from build123d import *
from build123d.topology import SkipClean

# Parameters (mm, degrees)
EXTRUDE_1_DEPTH          = 3
EXTRUDE_2_DEPTH          = 15
PATTERN_CIRCULAR_1_COUNT = 3
CUT_EXTRUDE_1_DEPTH      = 70.054326439


with BuildPart() as part:
    # Эскиз1 → Повернуть1 (revolve)
    with BuildSketch(Plane.XY, mode=Mode.PRIVATE) as revolve_1_sk:
        Polygon((0, 8), (0, 26.5), (10, 26.5), (10, 14), (40, 14), (40, 8), align=None)
    revolve(revolve_1_sk.sketch.rotate(Axis((0, 0, 0), (1, 0, 0)), 90), axis=Axis((0, 0, 0), (1, 0, 0)))

    # Эскиз2 → Бобышка-Вытянуть1 (add)
    with BuildSketch(Plane.ZY):
        with BuildLine():
            Line((22.9496732, 13.25), (14, 8.082903769))
            Line((14, 8.082903769), (14, -8.082903769))
            Line((14, -8.082903769), (22.9496732, -13.25))
            ThreePointArc((22.9496732, -13.25), (26.5, 0), (22.9496732, 13.25))
        make_face()
    extrude_1 = extrude(amount=EXTRUDE_1_DEPTH)

    # Эскиз3 → Бобышка-Вытянуть2 (add)
    with BuildSketch(Plane.ZY.offset(3)):
        with BuildLine():
            Line((25.037468802, 8.681886661), (14, 2.309401077))
            Line((14, 2.309401077), (14, -2.309401077))
            Line((14, -2.309401077), (25.037468802, -8.681886661))
            ThreePointArc((25.037468802, -8.681886661), (26.5, 0), (25.037468802, 8.681886661))
        make_face()
    extrude_2 = extrude(amount=EXTRUDE_2_DEPTH)

    # Круговой массив1: Бобышка-Вытянуть1, Бобышка-Вытянуть2 ×3 about axis
    with SkipClean():  # the faces are left unmerged after this step: merging them gives an invalid solid
        pattern_circular_1_axis = Axis((0, 0, 0), (1, 0, 0))
        add([extrude_1.rotate(pattern_circular_1_axis, i * 360 / PATTERN_CIRCULAR_1_COUNT) for i in range(1, PATTERN_CIRCULAR_1_COUNT)])
        add([extrude_2.rotate(pattern_circular_1_axis, i * 360 / PATTERN_CIRCULAR_1_COUNT) for i in range(1, PATTERN_CIRCULAR_1_COUNT)])

    # Эскиз4 → Вырез-Вытянуть1 (cut, through all)
    with SkipClean():  # the faces are left unmerged after this step: merging them gives an invalid solid
        with BuildSketch(Plane(origin=(40, 0, 0), x_dir=(0, 0, -1), z_dir=(1, 0, 0))):
            Polygon((-7.315063509, 7.670061659), (-2.984936491, 10.170061659), (2.165063509, 1.25), (-2.165063509, -1.25), align=None)
        extrude(amount=-CUT_EXTRUDE_1_DEPTH, mode=Mode.SUBTRACT)


solid = part.part
Source: CAD feature listing. Evaluate the final solid. Frame: model axes, mm. A direction names the side the tool comes from. Give positions to 0.01 mm unless a question says otherwise; leave off trailing zeros. Order: outer loops, then holes, each group sorted by start corner. A loop starts at its lowest first (then second) coordinate and runs counter-clockwise, first axis right, second up. Notation, with made-up numbers: (-3, 1) -> (13, 1) arc R19 ccw to (13, 38) -> close; hole circle Ø9 at (-15, 68). An arc over 180 degrees is marked (long way). Write item = value, one per line.
Q1. Pin query (flat end, axial travel): pin 1 (10 mm diameter, centred on y = -11, z = -17, fed in from -X); pin 2 (1.5 mm diameter, centred on y = -8.5, z = -19.5, fed in from +X); pin 3 (1 mm diameter, centred on x = -7.5, y = 11, fed in from +Z); pin 4 (4 mm diameter, centred on x = 8, z = 12, fed in from -Y). Return the tip coordinate at first contact, or that it passes through.
Data:
pin_1 = -18
pin_2 = 10
pin_3 = -8.08
pin_4 = -24.54
Q2. Cut plane D-D, the plane z = -12. Output: boundary loops of the cut face in (x, y), and give its area (3 significant figures).
Data:
outline = (-18, -23.63) -> (10, -23.63) -> (10, -7.21) -> (40, -7.21) -> (40, 7.21) -> (10, 7.21) -> (10, 23.63) -> (-18, 23.63) -> (-18, 12.7) -> (-3, 12.7) -> (-3, 9.24) -> (0, 9.24) -> (0, -9.24) -> (-3, -9.24) -> (-3, -12.7) -> (-18, -12.7) -> close
area = 1,320 mm^2
Q3. Material intervals for line 1 (Y direction, x = 19, z = 0); line 2 (X direction, y = 10, z = -3); line 3 (Z direction, x = 24.5, y = -6), sorted ascending. Write a range as from..to.
Data:
line_1 = -14..-8, 8..14
line_2 = 0..40
line_3 = -12.65..-5.29, 5.29..12.65
Q4. Pull-direction query (Z, two-part tool) for faces 1 (the face through (-7, 0, 14)), 2 (the face through (10, 11, 11)), 3 (the face through (25.2, 12.4, 6.5)), 4 (the face through (-1.48, -10.63, 18.41)); classes: released by +Z, released by -Z, zero draft, split by the parting line, or undercut.
Data:
face_1 = released by -Z
face_2 = zero draft
face_3 = split by the parting line
face_4 = undercut
Q5. Cut plane B-B, the plane x = -14. Output: boundary loops of the cut face in (y, z), and give its area (3 significant figures).
Data:
outline = (-26.02, -5) arc R26.5 ccw to (-17.34, -20.04) -> (-10.97, -9) -> (-13.28, -5) -> close; (-8.68, 25.04) -> (-2.31, 14) -> (2.31, 14) -> (8.68, 25.04) arc R26.5 ccw to start; (10.97, -9) -> (17.34, -20.04) arc R26.5 ccw to (26.02, -5) -> (13.28, -5) -> close
area = 415 mm^2
Q6. Cut plane C-C, the plane x = 27. Output: boundary loops of the cut face in (y, z), and give its area (3 significant figures).
Data:
outline = circle Ø28 at (0, 0); hole (5.33, 5.96) arc R8 ccw (long way) to (7.83, 1.63) -> (10.17, 2.98) -> (7.67, 7.32) -> close
area = 403 mm^2
Q7. Cut plane A-A, the plane y = 0. Output: boundary loops of the cut face in (x, z), and give its area (3 significant figures).
Data:
outline = (-18, 14) -> (0, 14) -> (0, 8) -> (40, 8) -> (40, 14) -> (10, 14) -> (10, 26.5) -> (-18, 26.5) -> close; (0, -26.5) -> (10, -26.5) -> (10, -14) -> (40, -14) -> (40, -8) -> (0, -8) -> close
area = 955 mm^2
Q8. Set-up query: faces 5 (the face through (-10.4, -5.45, 19.44)), 6 (the face through (-10.395, 5.54, 19.596)), 7 (the face through (-3, -8, 19)), 8 (the face through (-3, -13, -16)). Return all of +Z, -Z, +X, -X, +Y, -Y with unobstructed straight access to the full face (end or side cutting, diameter ignored); none if empty.
Data:
face_5 = -Z, -X, -Y
face_6 = -Z, -X, +Y
face_7 = -X, -Y
face_8 = -Z, -X
